Build history of the part. All positions in model axes, mm. A direction names the side the tool comes from. Coordinates: 2 decimals unless noted, no trailing zeros. Order: outer loops, then holes, each group sorted by start corner. A loop starts at its lowest first (then second) coordinate and runs counter-clockwise, first axis right, second up. Notation, with made-up numbers: (-29, 24) - (-25, 24) arc R30 cw to (-25, 50) - close; hole circle Ø11 at (-7.5, 7). An arc over 180 degrees is marked (long way). One line per item, written item: value.
from build123d import *

# Parameters (mm, degrees)
SKETCH1_W           = 56.0520382
SKETCH1_H           = 68.5
SKETCH1_R           = 1.5
SKETCH1_R_2         = 7.39
BOSS_EXTRUDE1_DEPTH = 6
SKETCH1_3_R         = 7.39
BOSS_EXTRUDE2_DEPTH = 5
CUT_EXTRUDE1_START  = -4
SKETCH2_R           = 1.95
SKETCH2_R_2         = 1.5
CUT_EXTRUDE1_DEPTH  = 4


with BuildPart() as part:
    # Sketch1 → Boss-Extrude1 (new body)
    # profile 1 of 2: a face of its own
    with BuildSketch(Plane(origin=(0, 0, 0), x_dir=(1, 0, 0), z_dir=(0, 1, 0))):
        with Locations((8.0260191, -14.25)):
            Rectangle(SKETCH1_W, SKETCH1_H)
        with Locations(Location((30.0520382, -30.0520382, 0), (0, 0, 270))):
            Circle(SKETCH1_R, mode=Mode.SUBTRACT)
        with Locations(Location((0, -42.5, 0), (0, 0, 270))):
            Circle(SKETCH1_R, mode=Mode.SUBTRACT)
        Circle(SKETCH1_R_2, mode=Mode.SUBTRACT)
    # profile 2 of 2: a face of its own
    with BuildSketch(Plane(origin=(0, 0, 0), x_dir=(1, 0, 0), z_dir=(0, 1, 0))):
        Circle(SKETCH1_R_2)
    extrude(amount=-BOSS_EXTRUDE1_DEPTH)

    # Sketch1_3 → Boss-Extrude2 (add)
    with BuildSketch(Plane(origin=(0, 0, 0), x_dir=(1, 0, 0), z_dir=(0, 1, 0))):
        with Locations(Location((0, 0, 0), (0, 0, 270))):
            Circle(SKETCH1_3_R)
    extrude(amount=BOSS_EXTRUDE2_DEPTH)

    # Sketch2 → Cut-Extrude1 (cut)
    # profile 1 of 2: a face of its own
    with BuildSketch(Plane.XZ.offset(6).offset(CUT_EXTRUDE1_START)):
        with Locations(Location((0, 42.5, 0), (0, 0, 270))):
            Circle(SKETCH2_R)
        with Locations(Location((0, 42.5, 0), (0, 0, 90))):
            Circle(SKETCH2_R_2, mode=Mode.SUBTRACT)
    # profile 2 of 2: a face of its own
    with BuildSketch(Plane.XZ.offset(6).offset(CUT_EXTRUDE1_START)):
        with Locations(Location((30.0520382, 30.0520382, 0), (0, 0, 270))):
            Circle(SKETCH2_R)
        with Locations(Location((30.0520382, 30.0520382, 0), (0, 0, 90))):
            Circle(SKETCH2_R_2, mode=Mode.SUBTRACT)
    extrude(amount=CUT_EXTRUDE1_DEPTH, mode=Mode.SUBTRACT)


solid = part.part
1. Band-saw the part on A-A, the plane z = 42.5. Give the cut face in (x, y).
Values found:
outline: (-20, -6) - (-1.95, -6) - (-1.95, -2) - (-1.5, -2) - (-1.5, 0) - (-20, 0) - close; (1.5, -2) - (1.95, -2) - (1.95, -6) - (36.05, -6) - (36.05, 0) - (1.5, 0) - close
2. Band-saw the part on C-C, the plane z = 0. Give the cut face in (x, y), and give its area (3 significant figures).
Values found:
outline: (-20, -6) - (36.05, -6) - (36.05, 0) - (7.39, 0) - (7.39, 5) - (-7.39, 5) - (-7.39, 0) - (-20, 0) - close
area: 410 mm2
3. Band-saw the part on B-B, the plane x = 0. Give the cut face in (y, z), and give its area (3 significant figures).
Values found:
outline: (-6, -20) - (0, -20) - (0, -7.39) - (5, -7.39) - (5, 7.39) - (0, 7.39) - (0, 41) - (-2, 41) - (-2, 40.55) - (-6, 40.55) - close; (-6, 44.45) - (-2, 44.45) - (-2, 44) - (0, 44) - (0, 48.5) - (-6, 48.5) - close
area: 463 mm2
4. Band-saw the part on D-D, the plane x = 22. Give the cut face in (y, z), and give its area (3 significant figures).
Values found:
outline: (-6, -20) - (0, -20) - (0, 48.5) - (-6, 48.5) - close
area: 411 mm2
5. Two-plate mould, pull along X, no slides. Class faces 3 (the face through (31.07, -0.99, 28.95)), 4 (the face through (-7.214, 2.465, -1.602)), 5 (the face through (8, -3, -20)), 6 (the face through (-20, -3, 15)): pulls with the +X half, pulls with the -X half, needs draft (parallel to the pull), parting line crosses it, or undercut.
Values found:
face 3: undercut
face 4: parting line crosses it
face 5: needs draft
face 6: pulls with the -X half
6. Probe line 1 along X through (y, z) = (-3, 42.5); line 2 along Z through (x, y) = (0, -1.35); line 3 along X through (y, z) = (-1, 42.5). List the from-to ranges inside material, lowest first.
Values found:
line 1: x = -20 to -1.95, 1.95 to 36.05
line 2: z = -20 to 41, 44 to 48.5
line 3: x = -20 to -1.5, 1.5 to 36.05
7. 3-axis set-ups, long thin cutter, end or side, ignore diameter. For faces 1 (the face through (8, -6, 14)), 2 (the face through (-0.75, -3.97, 40.7)): which of +Z, -Z, +X, -X, +Y, -Y reach the whole face in a straight line?
Values found:
face 1: +Z, -Z, +X, -X, -Y
face 2: -Y
8. Flat gauge pins, fed straight in: P1, Ø1, axis at x = 14.5, z = 7, coming from the +Y side; P2, Ø1.2, axis at x = 29, z = 29.5, coming from the -Y side; P3, Ø4, axis at x = 6.5, y = 4, coming from the -Z side. Where does each tip first touch, or does it go through?
Values found:
P1: stops at y = 0
P2: stops at y = -2
P3: stops at z = -5.86
